Here's how the part is built. I have some questions about the finished solid (model axes, mm). Face numbers are marked on the shaded views. A direction names the side the tool comes from. Coordinates: 2 decimals unless noted, no trailing zeros. Order: outer loops, then holes, each group sorted by start corner. A loop starts at its lowest first (then second) coordinate and runs counter-clockwise, first axis right, second up. Notation, with made-up numbers: (-25, 63.25) - (25, 63.25) arc R23 ccw to (25, 99.25) - close; hole circle Ø3 at (52, 32.25). An arc over 180 degrees is marked (long way). Answer in a Markdown table with one row per item. Add a question column.
Item 1: I want a section at B-B (x = 15). Please give me the cut outline in (y, z).
Item 2: Will these pins go through, and if not, where does the flat tip stop? pin 1 Ø3 at (y, z) = (3.5, 4) entering from +X; pin 2 Ø2 at (x, z) = (26.5, 4.5) entering from -Y; pin 3 Ø3 at (y, z) = (-2.5, 4.5) entering from +X.
Item 3: Thinking about a two-plate mould opening in Y: for the marked faces 3, 4, 5 and 6, which applies, +Y half, -Y half, draft (parallel to the pull), parting line (faces both ways), or undercut?
Item 4: I want a section at C-C (y = 24). Count the separate pieces of the cut face and the enclosed holes in it, plus the area to 3 significant figures.
Item 5: I want a section at A-A (z = 2.1). Please give me the cut outline in (x, y).
Item 6: On a 3-axis mill with a long thin cutter (end or side, diameter ignored), from which of +Z, -Z, +X, -X, +Y, -Y can I reach the whole of each face in a straight line? I mean the marked faces 1 and 2. Say none if no direction works.
Item 7: If I drill on line 1 along Y through (x, z) = (0, 2.4); line 2 along X through (y, z) = (23.5, 4.4) (1 decimal); line 3 along X through (y, z) = (24, 2), over which ranges is the centre line in solid material (lowest first)? Write a range as from..to.
Solid Edge part; units mm, degrees
sketch "Sketch1" plane through (0, 0, 0) normal (0, 0, 1) x (1, 0, 0)
  line L0 (-9, 22.6274) -> (-9, 0)
  line L1 (6.364, -6.364) -> (28.9914, 16.2635)
  line L2 (0, 31.6274) -> (22.6274, 31.6274)
  arc A0 (6.364, -6.364) -> (-9, 0) centre (0, 0) cw
  arc A1 (22.6274, 31.6274) -> (28.9914, 16.2635) centre (22.6274, 22.6274) cw
  arc A2 (-9, 22.6274) -> (0, 31.6274) centre (0, 22.6274) cw
  circle A3 centre (0, 0) radius 2.7
  circle A4 centre (0, 22.6274) radius 2.7
  circle A5 centre (22.6274, 22.6274) radius 2.7
extrude "Protrusion1" add sketch "Sketch1" along normal blind 6
sketch "Sketch2" plane through (11.3137, 11.3137, 6) normal (0, 0, 1) x (1, 0, 0)
  line L0 (2.364, -0.364) -> (24.7236, -0.364)
  arc A0 (0.364, -2.364) -> (2.364, -0.364) centre (2.364, -2.364) cw
  line L1 (0.364, -23.5521) -> (0.364, -2.364)
extrude "Cutout1" cut sketch "Sketch2" against normal through all material side at (24.8575, 10.8997, 6)
fillet "Round_1" radius 2 2 edges at (11.6777, -1.0503, 3) (23.6777, 10.9497, 3)
chamfer "Chamfer_1" distance 0.5 angle 45 3 edges at (-2.7, 0, 6) (-2.7, 22.6274, 6) (19.9274, 22.6274, 6)
properties material "ABS Plastic, medium impact"
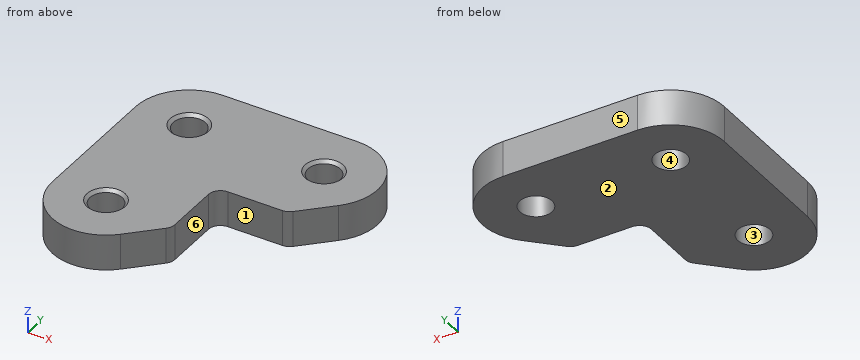
Values follow:
| question | item | result |
|---|---|---|
| 1 | outline | (10.95, 0) - (31.63, 0) - (31.63, 6) - (10.95, 6) - close |
| 2 | pin 1 | stops at x = 11.68 |
| 2 | pin 2 | stops at y = 12.77 |
| 2 | pin 3 | stops at x = 11.52 |
| 3 | face 3 | undercut |
| 3 | face 4 | undercut |
| 3 | face 5 | +Y half |
| 3 | face 6 | draft |
| 4 | separate pieces | 3 |
| 4 | enclosed holes | 0 |
| 4 | area | 186 mm^2 |
| 5 | outline | (-9, 0) arc R9 ccw to (6.36, -6.36) - (11.09, -1.64) arc R2 ccw to (11.68, -0.22) - (11.68, 8.95) arc R2 cw to (13.68, 10.95) - (22.85, 10.95) arc R2 ccw to (24.26, 11.54) - (28.99, 16.26) arc R9 ccw to (22.63, 31.63) - (0, 31.63) arc R9 ccw to (-9, 22.63) - close; hole circle Ø5.4 at (0, 0); hole circle Ø5.4 at (0, 22.63); hole circle Ø5.4 at (22.63, 22.63) |
| 6 | face 1 | +Z, -Z, +X, -Y |
| 6 | face 2 | -Z, +X, -X, +Y, -Y |
| 7 | line 1 | y = -9..-2.7, 2.7..19.93, 25.33..31.63 |
| 7 | line 2 | x = -9..-2.6, 2.6..20.1, 25.2..31.6 |
| 7 | line 3 | x = -8.89..-2.33, 2.33..20.3, 24.95..31.52 |
